Build history of the part. All positions in model axes, mm. A direction names the side the tool comes from. Round coordinates to 2 decimals unless told otherwise and drop trailing zeros. Loops run counter-clockwise (first coordinate to the right, second up) from the corner with the lowest first, then second, coordinate; pieces in that order, holes last. Notation, with made-up numbers: M 47,-6 L 92,-6 A27 ccw 92,19 Z; hole C 49,0.25 d7. An arc over 180 degrees is marked long. Write each question's results on one line, items separated by ' | '. Start each with the question number.
```python
from build123d import *

# Parameters (mm, degrees)
F0_R     = 26.8467875173
F1_DEPTH = 115
F3_DEPTH = 10
F5_R     = 5


# Not quite as in the source:
# - a feature of the source that left no trace in its solid (it failed there, or was rolled back) is left out


with BuildPart() as f1:
    # F0 (on Top) → F1 (new body)
    with BuildSketch(Plane.XY):
        Circle(F0_R)
        Polygon((-21.0732848254, 0), (-10.5366424127, 18.25), (10.5366424127, 18.25), (21.0732848254, 0), (10.5366424127, -18.25), (-10.5366424127, -18.25), align=None, mode=Mode.SUBTRACT)
    extrude(amount=F1_DEPTH)

    # F2 (on Top) → F3 (join)
    with BuildSketch(Plane.XY):
        Polygon((-40, 5), (-40, 0), (-40, -5), (-21.0732848254, -5), (-21.0732848254, 0), (-21.0732848254, 5), align=None)
        Polygon((0, 40), (-5, 40), (-5, 21.0732848254), (0, 21.0732848254), (5, 21.0732848254), (5, 40), align=None)
        Polygon((40, 0), (40, 5), (21.0732848254, 5), (21.0732848254, 0), (21.0732848254, -5), (40, -5), align=None)
        Polygon((0, -40), (5, -40), (5, -21.0732848254), (0, -21.0732848254), (-5, -21.0732848254), (-5, -40), align=None)
    extrude(amount=F3_DEPTH)

    # F5
    f5_edges = [f1.edges().sort_by_distance(p)[0] for p in [
        (0, 26.846788, 10),
        (-26.846788, 0, 10),
        (0, -26.846788, 10),
        (26.729101, 2.511007, 10),
        (26.729101, -2.511007, 10),
        (26.377073, -5, 5),
        (5, -26.377073, 5),
        (-5, -26.377073, 5),
        (-26.377073, -5, 5),
        (-26.377073, 5, 5),
        (-5, 26.377073, 5),
        (5, 26.377073, 5),
        (26.377073, 5, 5),
    ]]
    fillet(f5_edges, radius=F5_R)


solid = f1.part
```
Item 1: Tool access for faces 4 (the cylindrical face through (12.388, -23.818, 56.695)), 5 (the flat face through (15.879, -8.997, 56.695)), 6 (the flat face through (-35, -5, 5)), 7 (the flat face through (36, 0, 10)), 8 (the flat face through (5, -35, 5)): list every direction of +Z, -Z, +X, -X, +Y, -Y with a clear straight run to the whole face (end or side of a thin tool).
Item 2: Saw through at A-A, the plane z = 72.5. Give the cut face in (x, y).
Item 3: Mould opens along Y. For faces 1 (the flat face through (0, -18.25, 57)), 2 (the flat face through (-18, -6, 0)), 3 (the flat face through (35, 5, 5)) say: released by +Y, released by -Y, zero draft, split by the parting line, or undercut.
Item 4: Drill centre lines: line 1 along Y through (x, z) = (18, 31.5); line 2 along Y through (x, z) = (9.5, 11.5); line 3 along X through (y, z) = (17, 8). Where is each one in solid material? Low to high. Write a range as [from, to].
Item 5: Saw through at B-B, the plane x = 0. Give the cut face in (y, z).
Item 6: Saw through at C-C, the plane y = -34.5. Give the cut face in (x, z), then the cut area to 3 significant figures.
Item 7: Drop flat-ended pins along their axis: pin 1 (3 mm diameter, centred on x = 18.5, y = 15, fed in from -Z); pin 2 (3 mm diameter, centred on y = 9.5, z = 89.5, fed in from +X); pin 3 (5 mm diameter, centred on y = 33.5, z = 2.5, fed in from +X); pin 4 (3 mm diameter, centred on x = 35.5, z = 7.5, fed in from +Y). Give the stop position or say it passes through.
Working result:
1) face 4: +Z | face 5: +Z, -Z | face 6: +Z, -Z, -X, -Y | face 7: +Z, +X, +Y, -Y | face 8: +Z, -Z, +X, -Y
2) outline: C 0,0 d53.69; hole M -21.07,0 L -10.54,-18.25 L 10.54,-18.25 L 21.07,0 L 10.54,18.25 L -10.54,18.25 Z
3) face 1: undercut | face 2: zero draft | face 3: released by +Y
4) line 1: y = [-19.92, -5.32], [5.32, 19.92] | line 2: y = [-25.11, -18.25], [18.25, 25.11] | line 3: x = [-20.78, -11.26], [11.26, 20.78]
5) outline: M -40,0 L -18.25,0 L -18.25,115 L -26.85,115 L -26.85,15 A5 cw -31.85,10 L -40,10 Z; M 18.25,0 L 40,0 L 40,10 L 31.85,10 A5 cw 26.85,15 L 26.85,115 L 18.25,115 Z
6) outline: M -5,0 L 5,0 L 5,10 L -5,10 Z | area: 100 mm²
7) pin 1: stops at z = 0 | pin 2: stops at x = 25.63 | pin 3: stops at x = 5 | pin 4: stops at y = 5
